Autodesk Inventor part; units mm, degrees
ref_plane "YZ Plane" through (0, 0, 0) normal (1, 0, 0) x (0, 1, 0)
ref_plane "XZ Plane" through (0, 0, 0) normal (0, 1, 0) x (-1, 0, 0)
ref_plane "XY Plane" through (0, 0, 0) normal (0, 0, 1) x (1, 0, 0)
sketch "スケッチ1" plane through (0, 0, 0) normal (0, 0, 1) x (1, 0, 0)
  circle A0 centre (0, 0) radius 4.05
  circle A1 centre (0, 0) radius 6.05
  dimension "d0" = 8.1
  dimension "d1" = 2
extrude "押し出し1" add sketch "スケッチ1" against normal blind 8.1
sketch "スケッチ2" plane through (0, 0, -8.1) normal (0, 0, -1) x (-1, 0, 0)
  circle A0 centre (0, 0) radius 7.5
  circle A1 centre (0, 0) radius 7.5
  dimension "d10" = 15
extrude "押し出し2" add sketch "スケッチ2" along normal blind 9
sketch "スケッチ3" plane through (0, 0, 0) normal (0, 1, 0) x (-1, 0, 0)
  circle A0 centre (0, -12.6) radius 1.25
  line L0 (4.05, -8.1) -> (-4.05, -8.1)
  point P0 (0, 0)
  dimension "d6" = 2.5
  dimension "d7" = 4.5
extrude "押し出し3" cut sketch "スケッチ3" along normal through all both and the other way through all
fillet "フィレット1" radius 1 2 edges at (-6.05, 0, -8.1) (7.5, 0, -8.1)
fillet "フィレット2" radius 1 1 edges at (-6.05, 0, 0)
properties part number "parent_ver."
For this review, take the finished solid that the model builds, in its own axes (mm). A direction names the side the tool comes from. Coordinates: 2 decimals unless noted, no trailing zeros. Loops run counter-clockwise (first coordinate to the right, second up) from the corner with the lowest first, then second, coordinate; pieces in that order, holes last. Notation, with made-up numbers: (49.5, 86) - (105.5, 86) arc R27 cw to (105.5, 106) - close; hole circle Ø11 at (-21, 22). An arc over 180 degrees is marked (long way). Return JSON: item names as keys, results as strings.
Item 1: For faces 1 (the flat face through (0, 0, -17.1)), 2 (the cylindrical face through (-0.878, -3.954, -3.993)), list the 3-axis set-ups (+Z, -Z, +X, -X, +Y, -Y) from which the entire face can be reached by the end or side of a thin tool; tool diameter is ignored.
Determined:
{"face 1": "-Z, +X, -X, +Y, -Y", "face 2": "+Z"}
Item 2: Take a section at A-A (z = -4). Give the boundary of the cut face in (x, y).
Determined:
{"outline": "circle Ø12.1 at (0, 0); hole circle Ø8.1 at (0, 0)"}
Item 3: Insertion check: pin 1 (1.5 mm diameter, centred on x = 0, z = -12.6, fed in from -Y); pin 2 (4 mm diameter, centred on x = 2.5, z = -13.5, fed in from -Y); pin 3 (4 mm diameter, centred on x = 0.5, y = 1, fed in from +Z); pin 4 (3 mm diameter, centred on x = 2.5, z = -14, fed in from +Y). Each pin has a flat end and moves straight along its axis. Give the tip position at first contact, or say it passes through.
Determined:
{"pin 1": "passes through", "pin 2": "stops at y = -7.48", "pin 3": "stops at z = -8.1", "pin 4": "stops at y = 7.43"}
Item 4: Take a section at B-B (z = -13). Give the boundary of the cut face in (x, y).
Determined:
{"outline": "(-1.18, -7.41) - (-1.18, 7.41) arc R7.5 ccw to start; (1.18, -7.41) arc R7.5 ccw to (1.18, 7.41) - close"}
Item 5: Mouldability with a two-part tool opening along X and no side actions: class faces 3 (the flat face through (0, 0, -8.1)), 4 (the cylindrical face through (1.63, 7.32, -13)), 5 (the cylindrical face through (-0.577, -0.105, -11.491)), 6 (the flat face through (-4, 2, 0)) as pulls with the +X half, pulls with the -X half, needs draft (parallel to the pull), parting line crosses it, or undercut.
Determined:
{"face 3": "undercut", "face 4": "parting line crosses it", "face 5": "undercut", "face 6": "needs draft"}
Item 6: Take a section at C-C (z = -9.5). Give the boundary of the cut face in (x, y).
Determined:
{"outline": "circle Ø15 at (0, 0)"}
Item 7: For line 1 (Z direction, x = 0, y = -1.25); line 2 (Y direction, x = 2.5, z = -1.25); line 3 (Y direction, x = 1.25, z = -3.5), list the stretches that pass through material, from the lowest coordinate up.
Determined:
{"line 1": "z = -17.1 to -13.85, -11.35 to -8.1", "line 2": "y = -5.51 to -3.19, 3.19 to 5.51", "line 3": "y = -5.92 to -3.85, 3.85 to 5.92"}
